Input: part model. Units: mm. Frame: model coordinates. A direction names the side the tool comes from. Give positions to 0.01 mm unless a question says otherwise; leave off trailing zeros. Loops run counter-clockwise (first coordinate to the right, second up) from the corner with the lowest first, then second, coordinate; pieces in that order, holes last.
from build123d import *

# Parameters (mm, degrees)
SKETCH1_R           = 25
SKETCH1_R_2         = 0.85
BOSS_EXTRUDE1_DEPTH = 3.18
CUT_EXTRUDE1_DEPTH  = 36.498061919


with BuildPart() as part:
    # Sketch1 → Boss-Extrude1 (new body)
    with BuildSketch(Plane.XY):
        with Locations(Location((0, 0, 0), (0, 0, 180))):
            Circle(SKETCH1_R)
        with Locations(Location((0, 0, 0), (0, 0, 180))):
            Circle(SKETCH1_R_2, mode=Mode.SUBTRACT)
    extrude(amount=BOSS_EXTRUDE1_DEPTH)

    # Sketch2 → Cut-Extrude1 (cut, through all)
    with BuildSketch(Plane.XY.offset(3.18)):
        with BuildLine():
            ThreePointArc((-2.262973221, 3.114715428), (-1.189715428, 3.661567588), (0, 3.85))
            Line((0, 3.85), (0, 21.87181707))
            ThreePointArc((0, 21.87181707), (-6.758763172, 20.801334147), (-12.855931514, 17.694671707))
            Line((-12.855931514, 17.694671707), (-2.262973221, 3.114715428))
        make_face()
        with BuildLine():
            Line((12.855931514, 17.694671707), (2.262973221, 3.114715428))
            ThreePointArc((2.262973221, 3.114715428), (3.114715428, 2.262973221), (3.661567588, 1.189715428))
            Line((3.661567588, 1.189715428), (20.801334147, 6.758763172))
            ThreePointArc((20.801334147, 6.758763172), (17.694671707, 12.855931514), (12.855931514, 17.694671707))
        make_face()
        with BuildLine():
            ThreePointArc((-3.661567588, -1.189715428), (-3.85, 0), (-3.661567588, 1.189715428))
            Line((-3.661567588, 1.189715428), (-20.801334147, 6.758763172))
            ThreePointArc((-20.801334147, 6.758763172), (-21.87181707, 0), (-20.801334147, -6.758763172))
            Line((-20.801334147, -6.758763172), (-3.661567588, -1.189715428))
        make_face()
        with BuildLine():
            Line((20.801334147, -6.758763172), (3.661567588, -1.189715428))
            ThreePointArc((3.661567588, -1.189715428), (3.114715428, -2.262973221), (2.262973221, -3.114715428))
            Line((2.262973221, -3.114715428), (12.855931514, -17.694671707))
            ThreePointArc((12.855931514, -17.694671707), (17.694671707, -12.855931514), (20.801334147, -6.758763172))
        make_face()
        with BuildLine():
            ThreePointArc((0, -3.85), (-1.189715428, -3.661567588), (-2.262973221, -3.114715428))
            Line((-2.262973221, -3.114715428), (-12.855931514, -17.694671707))
            ThreePointArc((-12.855931514, -17.694671707), (-6.758763172, -20.801334147), (0, -21.87181707))
            Line((0, -21.87181707), (0, -3.85))
        make_face()
    extrude(amount=-CUT_EXTRUDE1_DEPTH, mode=Mode.SUBTRACT)


solid = part.part
(1) Mould query, pull axis X, two halves, no side actions, for faces 3 (the cylindrical face through (-23.846, -7.509, 1.568)), 4 (the flat face through (0.3, 5.2, 0)), 5 (the flat face through (7.634, 10.507, 1.612)), 6 (the cylindrical face through (0.18, 0.83, 1.57)). Classes: +X half, -X half, draft (parallel to the pull), parting line (faces both ways), or undercut.
Values follow:
face 3: parting line
face 4: draft
face 5: undercut
face 6: undercut
(2) Cut plane B-B (z = 1.15). Return the cut outline in (x, y).
Values follow:
outline: circle Ø50 at (0, 0); hole (-20.8, -6.76) - (-3.66, -1.19) arc R3.85 cw to (-3.66, 1.19) - (-20.8, 6.76) arc R21.87 ccw to start; hole (-12.86, -17.69) arc R21.87 ccw to (0, -21.87) - (0, -3.85) arc R3.85 cw to (-2.26, -3.11) - close; hole (-12.86, 17.69) - (-2.26, 3.11) arc R3.85 cw to (0, 3.85) - (0, 21.87) arc R21.87 ccw to start; hole circle Ø1.7 at (0, 0); hole (2.26, -3.11) - (12.86, -17.69) arc R21.87 ccw to (20.8, -6.76) - (3.66, -1.19) arc R3.85 cw to start; hole (2.26, 3.11) arc R3.85 cw to (3.66, 1.19) - (20.8, 6.76) arc R21.87 ccw to (12.86, 17.69) - close
(3) Cut plane A-A (y = 0). Return the cut outline in (x, z), and give its area (3 significant figures).
Values follow:
outline: (-25, 0) - (-21.87, 0) - (-21.87, 3.18) - (-25, 3.18) - close; (-3.85, 0) - (-0.85, 0) - (-0.85, 3.18) - (-3.85, 3.18) - close; (0.85, 0) - (25, 0) - (25, 3.18) - (0.85, 3.18) - close
area: 96.3 mm2
(4) Cut plane D-D (y = 5). Return the cut outline in (x, z).
Values follow:
outline: (-24.49, 0) - (-21.29, 0) - (-21.29, 3.18) - (-24.49, 3.18) - close; (-15.39, 0) - (-3.63, 0) - (-3.63, 3.18) - (-15.39, 3.18) - close; (0, 0) - (3.63, 0) - (3.63, 3.18) - (0, 3.18) - close; (15.39, 0) - (24.49, 0) - (24.49, 3.18) - (15.39, 3.18) - close
(5) Reachability of faces 1 (the cylindrical face through (3.1, 2.28, 1.61)), 2 (the flat face through (0.3, 5.2, 3.18)) from +Z, -Z, +X, -X, +Y, -Y: full face, straight path, thin tool, end or side. Return the list, or none.
Values follow:
face 1: +Z, -Z
face 2: +Z, +X, -X, +Y, -Y
(6) Cut plane C-C (x = 9). Return the cut outline in (y, z).
Values follow:
outline: (-23.32, 0) - (-12.39, 0) - (-12.39, 3.18) - (-23.32, 3.18) - close; (-2.92, 0) - (2.92, 0) - (2.92, 3.18) - (-2.92, 3.18) - close; (12.39, 0) - (23.32, 0) - (23.32, 3.18) - (12.39, 3.18) - close
(7) Ray query, probe 1 along Y at (x, z) = (3, 1.4); probe 2 along Y at (x, z) = (14.5, 1.3); probe 3 along X at (y, z) = (-12, 0.8). Return the intervals inside material, ascending.
Values follow:
probe 1: y = -24.82 to -4.13, -2.41 to 2.41, 4.13 to 24.82
probe 2: y = -20.37 to -16.37, -4.71 to 4.71, 16.37 to 20.37
probe 3: x = -21.93 to -8.72, 0 to 8.72, 18.29 to 21.93
(8) Pin query (flat end, axial travel): pin 1 Ø1.5 at (x, y) = (0, 0) entering from -Z; pin 2 Ø1.6 at (y, z) = (-13, 2) entering from -X; pin 3 Ø1 at (y, z) = (6.5, 1) entering from -X; pin 4 Ø1.6 at (y, z) = (11.5, 1) entering from -X. Return the tip coordinate at first contact, or that it passes through.
Values follow:
pin 1: passes through
pin 2: stops at x = -21.82
pin 3: stops at x = -24.27
pin 4: stops at x = -22.59
